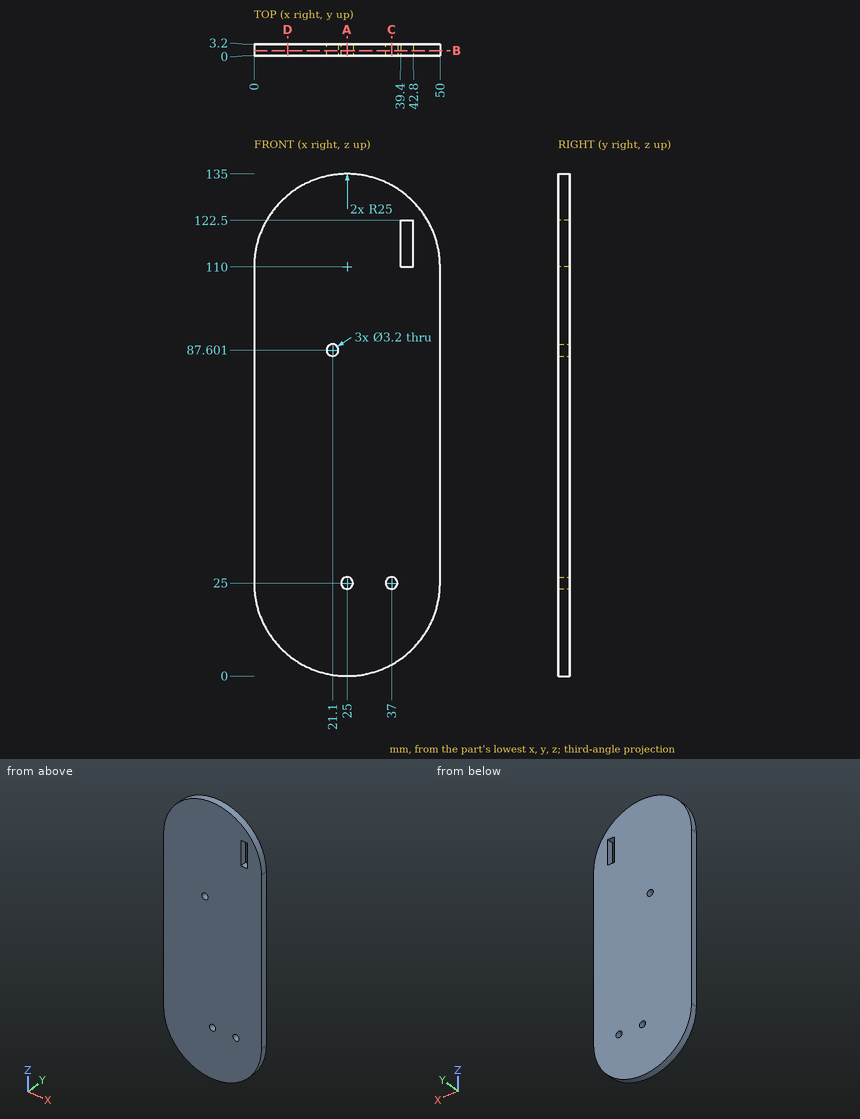
The figure shows three views and two pictorial views of one solid part (mm, origin at its lowest corner). Answer the questions. Round coordinates to 2 decimals unless told otherwise and drop trailing zeros. Write each loop counter-clockwise with the first axis right and the second up, starting at its lowest first coordinate (ties: lowest second). Pieces come first, ordered by that corner, then holes. Notation, with made-up numbers: (-11, 38) - (48, 38) arc R24 cw to (48, 49) - close; hole circle Ø11 at (-26, 65.25). An arc over 180 degrees is marked (long way). Use one line per item in the form item = value. Start each with the question number.
Item 1: Find the intervals of material crossed by line 1 (Z direction, x = 25, y = 1.35); line 2 (X direction, y = 0.25, z = 116.5); line 3 (Z direction, x = 33.5, y = 2.35), in increasing order. Write a range as [from, to].
Item 2: A cutting plane is placed at C-C (x = 37). Write down the section's boundary in (y, z).
Item 3: A cutting plane is placed at A-A (x = 25). Write down the section's boundary in (y, z), plus the area to 3 significant figures.
Item 4: A cutting plane is placed at B-B (y = 1.4). Write down the section's boundary in (x, z), plus the area to 3 significant figures.
Item 5: A cutting plane is placed at D-D (x = 9). Write down the section's boundary in (y, z), plus the area to 3 significant figures.
Item 6: Flat-ended cylindrical pins translate along their axes: pin 1 Ø1 at (x, y) = (41.5, 2) entering from +Z; pin 2 Ø3.5 at (x, z) = (25, 25) entering from -Y; pin 3 Ø1 at (y, z) = (1.5, 119) entering from -X. Find the tip coordinate at first contact, or state that the pin passes through.
The answers:
q1.line_1 = [0, 23.4], [26.6, 135]
q1.line_2 = [0.86, 39.4], [42.8, 49.14]
q1.line_3 = [1.49, 133.51]
q2.outline = (0, 3.07) - (3.2, 3.07) - (3.2, 23.4) - (0, 23.4) - close; (0, 26.6) - (3.2, 26.6) - (3.2, 131.93) - (0, 131.93) - close
q3.outline = (0, 0) - (3.2, 0) - (3.2, 23.4) - (0, 23.4) - close; (0, 26.6) - (3.2, 26.6) - (3.2, 135) - (0, 135) - close
q3.area = 422 mm^2
q4.outline = (0, 25) arc R25 ccw to (50, 25) - (50, 110) arc R25 ccw to (0, 110) - close; hole circle Ø3.2 at (21.1, 87.6); hole circle Ø3.2 at (25, 25); hole circle Ø3.2 at (37, 25); hole (39.4, 110) - (42.8, 110) - (42.8, 122.5) - (39.4, 122.5) - close
q4.area = 6,150 mm^2
q5.outline = (0, 5.79) - (3.2, 5.79) - (3.2, 129.21) - (0, 129.21) - close
q5.area = 395 mm^2
q6.pin_1 = 129.21
q6.pin_2 = 0
q6.pin_3 = 1.49
